Geometry check sheet. Reference: the model listing, model coordinates, mm. Round coordinates to 2 decimals unless told otherwise and drop trailing zeros. Order: outer loops, then holes, each group sorted by start corner. A loop starts at its lowest first (then second) coordinate and runs counter-clockwise, first axis right, second up. Notation, with made-up numbers: (4.5, 42) - (43.5, 42) arc R14 cw to (43.5, 67) - close; hole circle Ø6 at (-7, -6). An arc over 180 degrees is marked (long way). Answer as CSV lines item,"result". Start each with the question number.
```python
from build123d import *

# Parameters (mm, degrees)
SKETCH1_R           = 2.9337
BOSS_EXTRUDE1_DEPTH = 85.725


with BuildPart() as part:
    # Sketch1 → Boss-Extrude1 (new body)
    with BuildSketch(Plane.XY):
        with BuildLine():
            Line((-1.587500385, 6.349999904), (-3.666174594, 6.349999778))
            Line((-3.666174594, 6.349999778), (-4.70551159, 4.549815043))
            ThreePointArc((-4.70551159, 4.549815043), (-4.12444613, 2.38124975), (-6.293011423, 1.80018429))
            Line((-6.293011423, 1.80018429), (-7.332348419, -4.44e-07))
            Line((-7.332348419, -4.44e-07), (-6.293011205, -1.800185053))
            ThreePointArc((-6.293011205, -1.800185053), (-4.124445841, -2.38125025), (-4.705511038, -4.549815614))
            Line((-4.705511038, -4.549815614), (-3.666173825, -6.350000222))
            Line((-3.666173825, -6.350000222), (-1.587499615, -6.350000096))
            ThreePointArc((-1.587499615, -6.350000096), (2.89e-07, -4.7625), (1.587500385, -6.349999904))
            Line((1.587500385, -6.349999904), (3.666174594, -6.349999778))
            Line((3.666174594, -6.349999778), (4.70551159, -4.549815043))
            ThreePointArc((4.70551159, -4.549815043), (4.12444613, -2.38124975), (6.293011423, -1.80018429))
            Line((6.293011423, -1.80018429), (7.332348419, 4.44e-07))
            Line((7.332348419, 4.44e-07), (6.293011205, 1.800185053))
            ThreePointArc((6.293011205, 1.800185053), (4.124445841, 2.38125025), (4.705511038, 4.549815614))
            Line((4.705511038, 4.549815614), (3.666173825, 6.350000222))
            Line((3.666173825, 6.350000222), (1.587499615, 6.350000096))
            ThreePointArc((1.587499615, 6.350000096), (-2.89e-07, 4.7625), (-1.587500385, 6.349999904))
        make_face()
        Circle(SKETCH1_R, mode=Mode.SUBTRACT)
    extrude(amount=BOSS_EXTRUDE1_DEPTH)


solid = part.part
```
1. Thickness scan on probe 1 along Y at (x, z) = (0, 39); probe 2 along Y at (x, z) = (4.5, 52); probe 3 along X at (y, z) = (-5.5, 36). Record the ranges inside material, lowest first.
2. Section check A-A on x = 0. Record the boundary of the cut face in (y, z) (1 decimal), plus the area to 3 significant figures.
3. Draft check along Y on faces 1 (the face through (6.805, -0.913, 42.262)), 2 (the face through (4.19, 5.44, 42.26)), 3 (the face through (4.142, 2.351, 42.262)), 4 (the face through (-0.636, -2.864, 42.262)). Enter one of: released by +Y, released by -Y, zero draft, split by the parting line, or undercut.
4. Go/stop test with flat-tipped pins: pin 1 Ø1.5 at (y, z) = (2.5, 46) entering from -X; pin 2 Ø5.5 at (x, y) = (0, 0) entering from -Z; pin 3 Ø6 at (y, z) = (1, 63) entering from -X. Record where each tip stops, or that it passes through.
5. Section check C-C on y = 5.5. Record the boundary of the cut face in (x, z) (3 decimals), plus the area to 3 significant figures.
6. Section check D-D on x = 5.5. Record the boundary of the cut face in (y, z) (1 decimal).
Numbers:
1,probe 1,"y = -4.76 to -2.93, 2.93 to 4.76"
1,probe 2,"y = -4.91 to -4.41, -1.94 to 1.94, 4.41 to 4.91"
1,probe 3,"x = -4.16 to -1.34, 1.34 to 4.16"
2,outline,"(-4.8, 0) - (-2.9, 0) - (-2.9, 85.7) - (-4.8, 85.7) - close; (2.9, 0) - (4.8, 0) - (4.8, 85.7) - (2.9, 85.7) - close"
2,area,"314 mm2"
3,face 1,"released by -Y"
3,face 2,"released by +Y"
3,face 3,"undercut"
3,face 4,"undercut"
4,pin 1,"stops at x = -6.32"
4,pin 2,"passes through"
4,pin 3,"stops at x = -7.33"
5,outline,"(-4.157, 0) - (-1.341, 0) - (-1.341, 85.725) - (-4.157, 85.725) - close; (1.341, 0) - (4.157, 0) - (4.157, 85.725) - (1.341, 85.725) - close"
5,area,"483 mm2"
6,outline,"(-1.6, 0) - (1.6, 0) - (1.6, 85.7) - (-1.6, 85.7) - close"
